Geometry check sheet. Reference: the model listing, model coordinates, mm. A direction names the side the tool comes from. Give positions to 0.01 mm unless a question says otherwise; leave off trailing zeros. Order: outer loops, then holes, each group sorted by start corner. A loop starts at its lowest first (then second) coordinate and runs counter-clockwise, first axis right, second up. Notation, with made-up numbers: M -17.75,66 L 3.25,66 A22 ccw 3.25,100 Z; hole C 60,64 d9. An arc over 180 degrees is marked long. Put each result on its own line as item: value. Start each with the question number.
Q1. Section check B-B on x = 2.5. Record the cut outline in (y, z), then the cut area to 3 significant figures.
Q2. Section check D-D on y = -4. Record the cut outline in (x, z).
Q3. Access from +Z, -Z, +X, -X, +Y, -Y to the whole of each face (thin tool, end or side, straight path). Record for faces 1 (the flat face through (0, -3, -2)), 2 (the cylindrical face through (-2.404, -9.549, -3.135)), 3 (the flat face through (0, 0, 0)).
Q4. Section check A-A on z = 3.5. Record the cut outline in (x, y), then the cut area to 3 significant figures.
Q5. Section check C-C on y = -12. Record the cut outline in (x, z), then the cut area to 3 significant figures.
Q6. Go/stop test with flat-tipped pins: pin 1 (3 mm diameter, centred on x = -3.5, z = -3.5, fed in from +Y); pin 2 (5 mm diameter, centred on y = -9.5, z = -3.5, fed in from +X); pin 3 (5 mm diameter, centred on x = -1, y = -9.5, fed in from -Z). Record where each tip stops, or that it passes through.
Q7. Material ranges on L1, parallel to Y at x = 2, z = -1.25; L2, parallel to X at y = -11.5, z = 0; L3, parallel to X at y = -6.75, z = -1.5, recorded low to high.
```python
from build123d import *

# Parameters (mm, degrees)
F2_R = 1


with BuildPart() as f1:
    # F0 (on Right) → F1 (revolve)
    with BuildSketch(Plane.YZ):
        Polygon((-13, 0), (0, 0), (0, 1.5), (-3, 1.5), (-3, 4.45), (-6, 4.45), (-6, 3.95), (-13, 3.95), align=None)
    revolve(axis=Axis((0, -6.5, 0), (0, 1, 0)))

    # F2
    f2_edges = [f1.edges().sort_by_distance(p)[0] for p in [
        (0, 0, -1.5),
    ]]
    fillet(f2_edges, radius=F2_R)


solid = f1.part
```
Results found:
1. outline: M -13,-3.06 L -6,-3.06 L -6,-3.68 L -3,-3.68 L -3,3.68 L -6,3.68 L -6,3.06 L -13,3.06 Z
1. area: 64.9 mm^2
2. outline: C 0,0 d8.9
3. face 1: +Y
3. face 2: -Y
3. face 3: +Z, -Z, +X, -X, +Y
4. outline: M -2.75,-6 L -1.83,-6 L -1.83,-13 L 1.83,-13 L 1.83,-6 L 2.75,-6 L 2.75,-3 L -2.75,-3 Z
4. area: 42.1 mm^2
5. outline: C 0,0 d7.9
5. area: 49.0 mm^2
6. pin 1: stops at y = -3
6. pin 2: stops at x = 3.82
6. pin 3: stops at z = -3.95
7. L1: y = -13 to -3
7. L2: x = -3.95 to 3.95
7. L3: x = -3.65 to 3.65
